The listing builds one solid part. Answer for the finished solid, in the listing's coordinates (mm). Coordinates: 2 decimals unless noted, no trailing zeros. Order: outer loops, then holes, each group sorted by start corner. A loop starts at its lowest first (then second) coordinate and runs counter-clockwise, first axis right, second up. Notation, with made-up numbers: (3.5, 59) -> (46.5, 59) arc R16 cw to (46.5, 76) -> close; hole circle Ø3 at (5, -34). An arc over 180 degrees is marked (long way). Put each result on its own line as item: value. Start each with the question number.
```python
from build123d import *

# Parameters (mm, degrees)
SKETCH1_R           = 1.25
BOSS_EXTRUDE1_DEPTH = 8
SKETCH3_R           = 2.25
BOSS_EXTRUDE2_DEPTH = 1
CHAMFER3_SIZE       = 1
SKETCH4_R           = 0.5
CUT_EXTRUDE1_DEPTH  = 0.5
CUT_EXTRUDE2_DEPTH  = 0.25
CIRPATTERN1_COUNT   = 4
DRAFT1_ANGLE        = 2
FILLET4_R           = 0.2


with BuildPart() as part:
    # Sketch1 → Boss-Extrude1 (new body)
    with BuildSketch(Plane(origin=(0, 0, 0), x_dir=(1, 0, 0), z_dir=(0, 1, 0))):
        with Locations(Location((0, 0, 0), (0, 0, 270))):
            Circle(SKETCH1_R)
    extrude(amount=BOSS_EXTRUDE1_DEPTH)

    # Sketch3 → Boss-Extrude2 (add)
    with BuildSketch(Plane(origin=(0, 8, 0), x_dir=(1, 0, 0), z_dir=(0, 1, 0))):
        with Locations(Location((0, 0, 0), (0, 0, 270))):
            Circle(SKETCH3_R)
    extrude(amount=BOSS_EXTRUDE2_DEPTH)

    # Chamfer3
    chamfer3_edges = [part.edges().sort_by_distance(p)[0] for p in [
        (0, 8, -2.25),
    ]]
    chamfer(chamfer3_edges, length=CHAMFER3_SIZE - 0.0001)  # a hair under: the kernel refuses the full size

    # Sketch4 → Cut-Extrude1 (cut)
    with BuildSketch(Plane(origin=(0, 9, 0), x_dir=(1, 0, 0), z_dir=(0, 1, 0))):
        with Locations(Location((0, 0, 0), (0, 0, 270))):
            Circle(SKETCH4_R)
    extrude(amount=-CUT_EXTRUDE1_DEPTH, mode=Mode.SUBTRACT)

    # Sketch5 → Cut-Extrude2 (cut, symmetric)
    with BuildSketch(Plane.XY):
        Polygon((0.5, 8.5), (1.366025404, 9), (0.5, 9), (0.25, 9), (0.25, 8.5), align=None)
    cut_extrude2 = extrude(amount=CUT_EXTRUDE2_DEPTH, both=True, mode=Mode.SUBTRACT)

    # CirPattern1: Cut-Extrude2 ×4 about axis
    cirpattern1_axis = Axis((0, 0, 0), (0, 1, 0))
    for i in range(1, CIRPATTERN1_COUNT):
        add(cut_extrude2.rotate(cirpattern1_axis, i * 360 / CIRPATTERN1_COUNT), mode=Mode.SUBTRACT)

    # Draft1
    draft1_faces = [part.faces().sort_by_distance(p)[0] for p in [
        (-0.745512702, 8.822168784, -0.25),
    ]]
    draft(draft1_faces, Plane(origin=(-0.25, 0, 0), x_dir=(0, 0, 1), z_dir=(1, 0, 0)), DRAFT1_ANGLE)

    # Fillet4
    fillet4_edges = [part.edges().sort_by_distance(p)[0] for p in [
        (0.5, 8.5, 0),
        (1.366025404, 9, 0),
        (0, 8.5, -0.5),
        (0, 9, -1.366025404),
        (0, 9, 1.366025404),
        (-0.5, 8.5, 0.004365096),
        (-1.366025404, 9, 0.019486233),
    ]]
    fillet(fillet4_edges, radius=FILLET4_R)


solid = part.part
```
(1) This flat-tipped pin is pushed along its axis until it touches: P1, Ø1.5, axis at y = 5.5, z = 1, coming from the +X side. Where does it stop, or does it pass through?
(2) For a pull along Z with two mould halves and no side action, classify faces 1 (the flat face through (0, 0, 0)), 2 (the cylindrical face through (-1.22, 3.94, -0.27)), 3 (the flat face through (0, 8.5, 0)) as released by +Z, released by -Z, zero draft, split by the parting line, or undercut.
(3) The part is cut by section C-C on y = 6.5. Determine the outline of the cut face in (x, z).
(4) Find the intervals of material crossed by L1, parallel to Y at x = 0.4, z = -0.1; L2, parallel to X at y = 2.25, z = -0.05; L3, parallel to X at y = 8.75, z = 0.75, in increasing order.
Worked out:
1. P1: x = 1.22
2. face 1: zero draft
2. face 2: split by the parting line
2. face 3: undercut
3. outline: circle Ø2.5 at (0, 0)
4. L1: 0 to 8.5
4. L2: -1.25 to 1.25
4. L3: -1.85 to -0.25, 0.25 to 1.85
